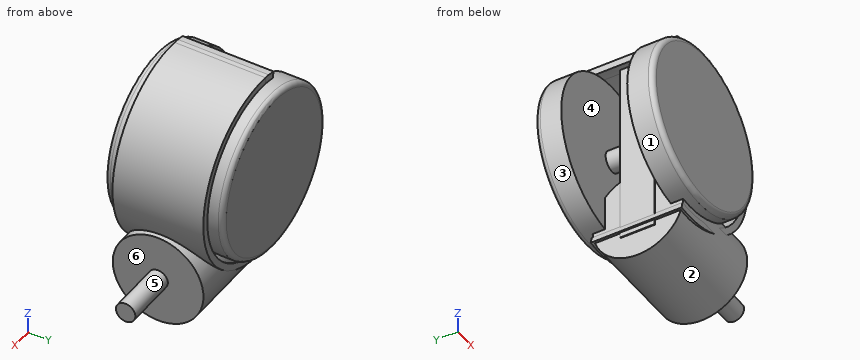
from build123d import *
from build123d import SkipClean  # not in build123d's __all__

# Parameters (mm, degrees)
F0_R      = 4
F1_DEPTH  = 12.7
F2_R      = 31.75
F3_DEPTH  = 10
F4_R      = 1.905
F6_W      = 15.24
F6_H      = 6.6250320524
F7_DEPTH  = 71.12
F9_W      = 1.8474994206
F9_H      = 34.9828377366
F10_DEPTH = 2.54
F11_ANGLE = 8
F12_ANGLE = 193
F13_R     = 3.75
F14_DEPTH = 20.32
F15_R     = 17.4624022324
F16_DEPTH = 40


with BuildPart() as f1:
    # F0 (on Front) → F1 (new body)
    with BuildSketch(Plane.XZ):
        with Locations((-55.9084378183, 37.7567484975)):
            Circle(F0_R)
    extrude(amount=F1_DEPTH)

    # F2 (on face) → F3 (join)
    with BuildSketch(Plane.XZ.offset(12.7)):
        with Locations((-55.9084378183, 37.7567484975)):
            Circle(F2_R)
    extrude(amount=F3_DEPTH)

    # F4
    f4_edges = [f1.edges().sort_by_distance(p)[0] for p in [
        (-87.658438, -22.7, 37.756748),
    ]]
    fillet(f4_edges, radius=F4_R)

    # F5: F1 across plane


with BuildPart() as f1_1:
    add(f1.part, clean=False)
    add(f1.part.mirror(Plane.XZ), clean=False)

    # F6 (on Top) → F7 (join)
    with BuildSketch(Plane.XY):
        with Locations((-53.0349581492, 3.3125160262)):
            Rectangle(F6_W, F6_H)
    extrude(amount=F7_DEPTH)

    # F8: F1 across plane


with BuildPart() as f1_2:
    add(f1_1.part, clean=False)
    add(f1_1.part.mirror(Plane.XZ), clean=False)

    # F9 (on face) → F10 (join)
    with BuildSketch(Plane.XY.offset(71.12)):
        with Locations((-59.7312084389, 0.1775659621)):
            Rectangle(F9_W, F9_H)
    extrude(amount=F10_DEPTH)

    # F10_face (on face) → F11 (revolve)
    with BuildSketch(Plane(origin=(-58.8074587286, 0.1775659621, 72.39), x_dir=(0, 1, 0), z_dir=(1, 0, 0))):
        Polygon((-17.4914188683, 1.27), (-17.4914188683, -1.27), (-6.8025980145, -1.27), (6.4474660903, -1.27), (17.4914188683, -1.27), (17.4914188683, 1.27), align=None)
    revolve(axis=Axis((-55.9084378183, -22.7, 37.7567484975), (0, -1, 0)), revolution_arc=F11_ANGLE)

    # F10_face (on face) → F12 (revolve)
    with BuildSketch(Plane(origin=(-58.8074587286, 0.1775659621, 72.39), x_dir=(0, 1, 0), z_dir=(1, 0, 0))):
        Polygon((-17.4914188683, 1.27), (-17.4914188683, -1.27), (-6.8025980145, -1.27), (6.4474660903, -1.27), (17.4914188683, -1.27), (17.4914188683, 1.27), align=None)
    with SkipClean():  # cleaning this boolean's faces spoils the solid; the shape is the same uncleaned
        revolve(axis=Axis((-55.9084378183, -22.7, 37.7567484975), (0, 1, 0)), revolution_arc=F12_ANGLE)



with BuildPart() as f14:
    # F13 (on Right) → F14 (new body)
    with BuildSketch(Plane.YZ):
        with Locations((0, 7.5903639288)):
            Circle(F13_R)
    extrude(amount=-F14_DEPTH)


with BuildPart() as f1_3:
    add(f1_2.part, clean=False)

    with SkipClean():  # cleaning this boolean's faces spoils the solid; the shape is the same uncleaned
        add(f14.part)  # F16 merges F14
    # F15 (on face) → F16 (join)
    with BuildSketch(Plane(origin=(-20.32, 0, 0), x_dir=(0, -1, 0), z_dir=(-1, 0, 0))):
        with Locations((0, 7.5903639288)):
            Circle(F15_R)
    with SkipClean():  # cleaning this boolean's faces spoils the solid; the shape is the same uncleaned
        extrude(amount=F16_DEPTH)


solid = f1_3.part
Design review of the part built by this model. Coordinates are the model's own, in mm. Face numbers are marked on the shaded views. A direction names the side the tool comes from. Round coordinates to 2 decimals unless told otherwise and drop trailing zeros. Write each loop counter-clockwise with the first axis right and the second up, starting at its lowest first coordinate (ties: lowest second). Pieces come first, ordered by that corner, then holes. Notation, with made-up numbers: (-28, -39) -> (-7, -39) arc R14 ccw to (-7, -15) -> close; hole circle Ø4 at (71.5, -40). An arc over 180 degrees is marked (long way). One line per item, written item: value. Start each with the question number.
Q1. Tool access review of the marked faces 1, 2 and 3: name each direction out of +Z, -Z, +X, -X, +Y, -Y from which nothing blocks a thin tool from reaching the whole face with its end or side.
Q2. Add section C-C (z = 21.5). State how many separate pieces and enclosed holes the cut face has, then the cut area to 3 significant figures.
Q3. The part is to be moulded in two halves that separate along Y. For the marked faces 4, 5 and 6, say which applies: pulls with the +Y half, pulls with the -Y half, needs draft (parallel to the pull), parting line crosses it, or undercut.
Q4. Add section A-A (y = 10). Give the boundary of the cut face in (x, z), then the cut area to 3 significant figures.
Q5. Insertion check: P1, Ø5.5, axis at y = -13, z = 13, coming from the -X side; P2, Ø1.5, axis at y = -5, z = -0.5, coming from the +X side; P3, Ø5, axis at y = 6.5, z = 10, coming from the -X side; P4, Ø1.5, axis at x = -72, z = 9, coming from the +Y side. Each pin has a flat end and moves straight along its axis. Give the tip position at first contact, or say it passes through.
Q6. To check wall thickness, follow probe 1 along Y at (x, z) = (-50, 30.5); probe 2 along Y at (x, z) = (-29.5, 28); probe 3 along Z at (x, y) = (-57.5, -10.5). State the ranges of each line that lie inside material, in increasing order.
Q7. Add section D-D (y = 19). Give the boundary of the cut face in (x, z), then the cut area to 3 significant figures.
Q8. Add section B-B (y = 0). Give the boundary of the cut face in (x, z), then the cut area to 3 significant figures.
Response:
1. face 1: -Y
1. face 2: none
1. face 3: +Y
2. separate pieces: 3
2. enclosed holes: 0
2. area: 1,980 mm^2
3. face 4: undercut
3. face 5: parting line crosses it
3. face 6: needs draft
4. outline: (-63.78, 72.91) -> (-63.42, 70.39) arc R33.49 cw to (-26.41, 21.91) -> (-60.32, 21.91) -> (-60.32, 4.56) arc R33.49 cw to (-60.59, 4.6) -> (-61.16, 2.12) arc R36.02 ccw to (-60.32, 2.01) -> (-60.32, -6.73) -> (-20.32, -6.73) -> (-20.32, 21.91) -> (-23.56, 21.91) arc R36.02 ccw to (-58.81, 73.66) -> (-60.65, 73.66) -> (-60.65, 73.46) arc R36.02 ccw to start; circle Ø8 at (-55.91, 37.76)
4. area: 1,400 mm^2
5. P1: stops at x = -78.79
5. P2: stops at x = -20.32
5. P3: stops at x = -60.65
5. P4: passes through
6. probe 1: y = -22.7 to -12.7, -6.63 to 6.63, 12.7 to 22.7
6. probe 2: y = -22.7 to -12.7, 12.7 to 22.7
6. probe 3: z = -6.36 to 21.54, 34.09 to 41.43, 71.21 to 73.74
7. outline: circle Ø63.5 at (-55.91, 37.76)
7. area: 3,170 mm^2
8. outline: (-63.78, 72.91) -> (-63.42, 70.39) arc R33.49 cw to (-60.65, 70.91) -> (-60.65, 4.31) -> (-61.16, 2.12) arc R36.02 ccw to (-60.65, 2.05) -> (-60.65, 0) -> (-60.32, 0) -> (-60.32, -9.87) -> (-20.32, -9.87) -> (-20.32, 3.84) -> (0, 3.84) -> (0, 11.34) -> (-20.32, 11.34) -> (-20.32, 25.05) -> (-22.2, 25.05) arc R36.02 ccw to (-58.81, 73.66) -> (-60.65, 73.66) -> (-60.65, 73.46) arc R36.02 ccw to start; hole (-58.81, 71.12) -> (-53.01, 71.12) arc R33.49 ccw to start; hole (-45.41, 25.05) -> (-24.92, 25.05) arc R33.49 ccw to (-45.41, 69.56) -> close
8. area: 2,450 mm^2
